The listing builds one solid part. Answer for the finished solid, in the listing's coordinates (mm). Coordinates: 2 decimals unless noted, no trailing zeros. Loops run counter-clockwise (first coordinate to the right, second up) from the corner with the lowest first, then second, coordinate; pieces in that order, holes last. Notation, with made-up numbers: (61, -2) - (99, -2) arc R8 cw to (99, 4) - close; hole circle Ø6 at (-8.5, 28.5). An arc over 180 degrees is marked (long way). Put each result on its own line as item: value.
```python
from build123d import *

# Parameters (mm, degrees)
SKETCH1_R           = 2
BOSS_EXTRUDE1_DEPTH = 60
SKETCH2_W           = 4
SKETCH2_H           = 40
BOSS_EXTRUDE2_DEPTH = 2.54
SKETCH3_W           = 4
SKETCH3_H           = 40
BOSS_EXTRUDE3_DEPTH = 2.54
SKETCH4_W           = 4.044012612
SKETCH4_H           = 65.108603045
BOSS_EXTRUDE4_DEPTH = 2.54


with BuildPart() as part:
    # Sketch1 → Boss-Extrude1 (new body)
    with BuildSketch(Plane(origin=(0, 0, 0), x_dir=(1, 0, 0), z_dir=(0, 1, 0))):
        Circle(SKETCH1_R)
    extrude(amount=BOSS_EXTRUDE1_DEPTH)

    # Sketch2 → Boss-Extrude2 (add)
    with BuildSketch(Plane.XZ):
        with Locations((0, 18)):
            Rectangle(SKETCH2_W, SKETCH2_H)
    extrude(amount=BOSS_EXTRUDE2_DEPTH)

    # Sketch3 → Boss-Extrude3 (add)
    with BuildSketch(Plane(origin=(0, 60, 0), x_dir=(1, 0, 0), z_dir=(0, 1, 0))):
        with Locations((0, -18)):
            Rectangle(SKETCH3_W, SKETCH3_H)
    extrude(amount=BOSS_EXTRUDE3_DEPTH)

    # Sketch4 → Boss-Extrude4 (add)
    with BuildSketch(Plane.XY.offset(38)):
        with Locations((0, 29.86519958)):
            Rectangle(SKETCH4_W, SKETCH4_H)
    extrude(amount=BOSS_EXTRUDE4_DEPTH)


solid = part.part
```
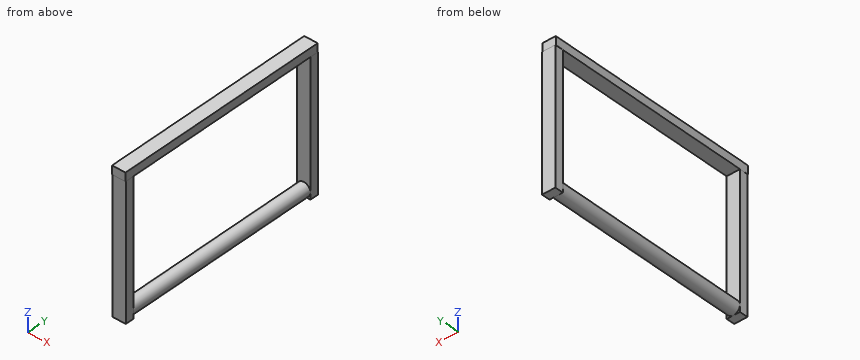
1) Each of these flat-tipped pins is pushed along its axis until it touches: pin 1 (3 mm diameter, centred on y = 62, z = 13, fed in from +X); pin 2 (2 mm diameter, centred on x = -0.5, z = -1, fed in from -Y); pin 3 (3 mm diameter, centred on y = -2, z = 25.5, fed in from -X). Where does it stop, or does it pass through?
Found:
pin 1: stops at x = 2
pin 2: stops at y = -2.54
pin 3: stops at x = -2
2) The part is cut by section B-B (z = 21.5). Give the vertices of the cut face in (x, y), and give its area (3 significant figures).
Found:
outline: (-2, -2.54) - (2, -2.54) - (2, 0) - (-2, 0) - close; (-2, 60) - (2, 60) - (2, 62.54) - (-2, 62.54) - close
area: 20.3 mm^2
3) The part is cut by section C-C (x = -0.9). Give the vertices of the cut face in (y, z).
Found:
outline: (-2.69, 38) - (-2.54, 38) - (-2.54, -2) - (0, -2) - (0, -1.79) - (60, -1.79) - (60, -2) - (62.54, -2) - (62.54, 38) - (62.42, 38) - (62.42, 40.54) - (-2.69, 40.54) - close; hole (0, 1.79) - (60, 1.79) - (60, 38) - (0, 38) - close
4) The part is cut by section A-A (y = 56.5). Give the vertices of the cut face in (x, z).
Found:
outline: (-2.02, 38) - (2.02, 38) - (2.02, 40.54) - (-2.02, 40.54) - close; circle Ø4 at (0, 0)
5) Straight lines are drawn through the part: L1, parallel to Y at x = -1.85, z = 23.5; L2, parallel to Z at x = -0.2, y = 41; L3, parallel to Z at x = 1.4, y = 35. For each, find the intervals that lie inside material, in ascending order. Write a range as [from, to].
Found:
L1: y = [-2.54, 0], [60, 62.54]
L2: z = [-1.99, 1.99], [38, 40.54]
L3: z = [-1.43, 1.43], [38, 40.54]
